Can you work these out from the model? Positions are in its coordinate system, mm. Face numbers are marked on the shaded views. Coordinates: 2 decimals unless noted, no trailing zeros. Write each loop counter-clockwise with the first axis right and the second up, starting at its lowest first coordinate (ties: lowest second). Pieces come first, ordered by that corner, then holes. Notation, with made-up numbers: (79, 59) -> (92, 59) arc R35 cw to (92, 91) -> close; hole circle Ø2 at (0, 33.25). An arc over 180 degrees is marked (long way). Use one line per item in the form item = value.
Autodesk Inventor part; units mm, degrees
ref_plane "YZ Plane" through (0, 0, 0) normal (1, 0, 0) x (0, 1, 0)
ref_plane "XZ Plane" through (0, 0, 0) normal (0, 1, 0) x (-1, 0, 0)
ref_plane "XY Plane" through (0, 0, 0) normal (0, 0, 1) x (1, 0, 0)
sketch "Эскиз1" plane through (0, 0, 0) normal (0, 1, 0) x (-1, 0, 0)
  circle A0 centre (0.1295, 0.2019) radius 7
  circle A1 centre (-6.8705, 7.2019) radius 1.5
  circle A2 centre (7.1295, 7.2019) radius 1.5
  circle A3 centre (7.1295, -6.7981) radius 1.5
  circle A4 centre (-6.8705, -6.7981) radius 1.5
  line L0 (-6.8705, -10.8093) -> (-6.8705, 13.8282) construction
  line L1 (14.3213, 7.2019) -> (-16.097, 7.2019) construction
  line L2 (7.1295, -11.068) -> (7.1295, 16.1729) construction
  arc A5 (6.5047, 14.6631) -> (7.1295, 16.1729) centre (4.9928, 16.1729) ccw construction
  line L3 (12.5583, -6.7981) -> (-15.6188, -6.7981) construction
  circle A6 centre (7.1295, 7.2019) radius 2.8995
  circle A7 centre (-6.8705, 7.2019) radius 2.8995
  circle A8 centre (-6.8705, -6.7981) radius 2.8995
  circle A9 centre (7.1295, -6.7981) radius 2.8995
  arc A10 (0.5599, -6.4772) -> (-0.2768, -6.4772) centre (0.1416, -8.4329) ccw
  line L4 (5.6295, -6.7981) -> (0.1295, -6.7981)
  line L5 (7.1295, -5.2981) -> (7.1295, 0.2019)
  line L6 (7.1295, 5.7019) -> (7.1295, 0.2019)
  line L7 (5.6295, 7.2019) -> (-5.3705, 7.2019)
  line L8 (-6.8705, 5.7019) -> (-6.8705, -5.2981)
  line L9 (-5.3705, -6.7981) -> (0.1295, -6.7981)
  circle A11 centre (0.1295, 0.2019) radius 8.3995
  circle A12 centre (0.1295, 0.2019) radius 6
  point P0 (-3.971, 7.2019)
  point P1 (-6.8705, 4.3024)
  point P2 (-6.8705, -3.8986)
  point P3 (-3.971, -6.7981)
  point P4 (4.23, -6.7981)
  point P5 (7.1295, -3.8986)
  point P6 (7.1295, 4.3024)
  point P7 (4.23, 7.2019)
  point P8 (4.2478, 7.5225)
  point P9 (-3.9888, 7.5225)
  point P10 (-7.1911, 4.3202)
  point P11 (-7.1911, -3.9164)
  point P12 (-3.9888, -7.1187)
  point P13 (4.2478, -7.1187)
  point P14 (7.4501, -3.9164)
  point P15 (7.4501, 4.3202)
  dimension "d23" = 14
  dimension "d24" = 3
  dimension "d25" = 3
  dimension "d26" = 3
  dimension "d27" = 3
  dimension "d28" = 2
  dimension "d40" = 12
extrude "Выдавливание1" add sketch "Эскиз1" along normal blind 3 contours L5 A9 A0 | L6 A6 A11 A9 L5 | A0 A6 L6 | A0 L7 A6 | A6 L7 A11 L6 | A9 L4 A0 | A9 L5 A11 L4 | A9 A11 L5 | L6 A11 A6 | L7 A7 A11 A6 | A0 A7 L7 | A6 A11 L7 | L9 A8 A0 | L4 A9 A11 A8 L9 | L4 A11 A9 | A9 A11 L4 A3 L5 | L5 A3 A11 | A11 L6 A2 L7 A6 | A11 A2 L6 | A0 L8 A7 | A7 L8 A11 L7 | L7 A11 A7 | L7 A2 A11 | A8 L8 A0 | A8 L9 A11 L8 | A8 A11 L9 | A11 A3 L4 | L8 A8 A11 A7 | A7 A11 L8 | A11 L7 A1 L8 A7 | A11 A1 L7 | L8 A11 A8 | A8 A11 L8 A4 L9 | L9 A4 A11 | L8 A1 A11 | A11 A4 L8
extrude "Выдавливание3" add sketch "Эскиз1" along normal up to surface (3 mm away) contours A0
fillet "Сопряжение грани1" radius 5 2 edges at (-4.2478, 1.5, 7.5225) (-7.4501, 1.5, 4.3202)
fillet "Сопряжение грани2" radius 5 2 edges at (3.9888, 1.5, 7.5225) (7.1911, 1.5, 4.3202)
fillet_without_effect "Сопряжение грани3"
fillet "Сопряжение грани4" radius 5 2 edges at (7.1911, 1.5, -3.9164) (3.9888, 1.5, -7.1187)
fillet "Сопряжение грани5" radius 5 2 edges at (-4.2478, 1.5, -7.1187) (-7.4501, 1.5, -3.9164)
fillet_without_effect "Сопряжение грани6"
fillet_without_effect "Сопряжение грани7"
fillet_without_effect "Сопряжение грани8"
properties part number "крепление подшипника_1_CPY"
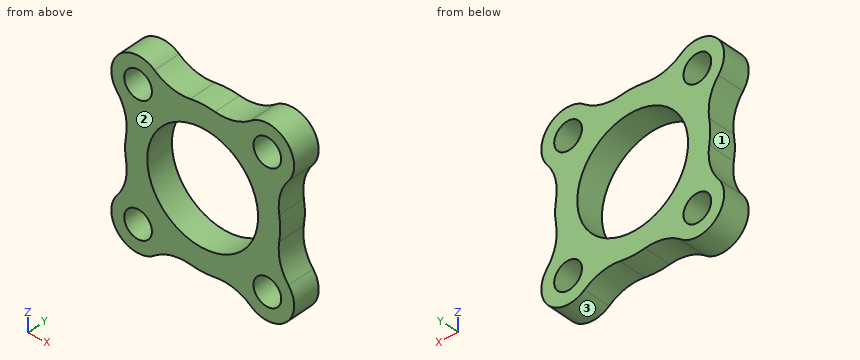
Q1. Suppose I cut it at D-D (z = 7.75). Write out the boundary of the cut face in (x, y), then the cut area to 3 significant figures.
Return value:
outline = (-9.98, 0) -> (-8.53, 0) -> (-8.53, 3) -> (-9.98, 3) -> close; (-5.73, 0) -> (5.47, 0) -> (5.47, 3) -> (-5.73, 3) -> close; (8.27, 0) -> (9.72, 0) -> (9.72, 3) -> (8.27, 3) -> close
area = 42.3 mm2
Q2. Suppose I cut it at A-A (x = 0). Write out the boundary of the cut face in (y, z).
Return value:
outline = (0, -8.2) -> (3, -8.2) -> (3, -5.8) -> (0, -5.8) -> close; (0, 6.2) -> (3, 6.2) -> (3, 8.6) -> (0, 8.6) -> close
Q3. Will this pin go through, and if not, where does the flat tip stop? pin 1 (1 mm diameter, centred on x = 0.5, y = 0.5, fed in from -Z).
Return value:
pin_1 = -8.2
Q4. If I drill on line 1 (Z direction, x = 8, y = 1.3); line 2 (Z direction, x = -6.25, y = 0.3); line 3 (X direction, y = 2.6, z = 6.25), over which ranges is the centre line in solid material (lowest first)? Write a range as from..to.
Return value:
line_1 = -9.47..-7.79, -5.81..6.21, 8.19..9.87
line_2 = -9.56..-8.01, -5.58..5.99, 8.42..9.96
line_3 = -9.87..-8.29, -5.97..5.71, 8.03..9.61
Q5. Thinking about a two-plate mould opening in X: for the marked faces 1, 2 and 3, which applies, released by +X, released by -X, zero draft, split by the parting line, or undercut?
Return value:
face_1 = released by -X
face_2 = zero draft
face_3 = undercut
Q6. Suppose I cut it at B-B (z = -7.25). Write out the boundary of the cut face in (x, y), then the cut area to 3 significant figures.
Return value:
outline = (-9.99, 0) -> (-8.56, 0) -> (-8.56, 3) -> (-9.99, 3) -> close; (-5.7, 0) -> (5.44, 0) -> (5.44, 3) -> (-5.7, 3) -> close; (8.3, 0) -> (9.73, 0) -> (9.73, 3) -> (8.3, 3) -> close
area = 42.0 mm2
Q7. Suppose I cut it at C-C (y = 2). Give the number of separate pieces and of enclosed holes in the cut face, then the cut area to 3 significant figures.
Return value:
separate_pieces = 1
enclosed_holes = 5
area = 181 mm2
